Verification items for the finished model (mm, model axes). A direction names the side the tool comes from. Give positions to 0.01 mm unless a question says otherwise; leave off trailing zeros. Order: outer loops, then holes, each group sorted by start corner. A loop starts at its lowest first (then second) coordinate and runs counter-clockwise, first axis right, second up. Notation, with made-up numbers: (39, 80.5) -> (91, 80.5) arc R13 cw to (91, 98.5) -> close; hole circle Ø3 at (12, 55.5). An arc over 180 degrees is marked (long way). Return JSON: item names as keys, results as strings. Group by question number.
(1) Cross-section at A-A on y = -11.5. State how many separate pieces and enclosed holes the cut face has, then the cut area to 3 significant figures.
(2) Thickness scan on line 1 along Z through (x, y) = (-10, -8.25); line 2 along Y through (x, z) = (5.5, 5); line 3 along X through (y, z) = (-8.5, 3.5). Record the ranges inside material, lowest first.
(3) Cross-section at B-B on x = 9. Enter the section's corners in (y, z), then the cut area to 3 significant figures.
(4) Depth check by flat-ended pin: pin 1 Ø4 at (x, z) = (9.5, 0.5) entering from +Y; pin 2 Ø5 at (x, y) = (5, -5.5) entering from -Z; pin 3 Ø0.8 at (x, z) = (7.5, -0.5) entering from -Y; pin 4 Ø7 at (x, z) = (-8, -0.5) entering from -Y. Enter the tip coordinate at first touch or a pass-through.
(5) Cross-section at D-D on y = -6. Enter the section's corners in (x, z) (3 decimals), then the cut area to 3 significant figures.
(6) Cross-section at C-C on z = 0. Enter the section's corners in (x, y), then the cut area to 3 significant figures.
(7) Release check for a two-part mould opening along X. For faces 4 (the face through (4.5, -6.4, -1.7)), 5 (the face through (10, -7, -0.8)), 6 (the face through (12.2, -7, -2)) record: pulls with the +X half, pulls with the -X half, needs draft (parallel to the pull), parting line crosses it, or undercut.
(8) Tool access check on faces 1 (the face through (0, -3, 5)), 2 (the face through (-11, -7, 3.175)), 3 (the face through (8.342, -0.456, 0.355)). Record the directions out of +Z, -Z, +X, -X, +Y, -Y that give a thin tool (end or side, any length) a straight path to the whole face; none if there is none.
from build123d import *

# Parameters (mm, degrees)
SKETCH_2_R          = 0.75
EXTRUDE_1_DEPTH     = 1.5
CUT_EXTRUDE_1_DEPTH = 1.5
EXTRUDE_2_DEPTH     = 2.8
SKETCH_5_R          = 0.3
EXTRUDE_3_DEPTH     = 4.6


with BuildPart() as part:
    # 草图1 → 旋转1 (revolve)
    with BuildSketch(Plane.XY, mode=Mode.PRIVATE) as revolve_1_sk:
        Polygon((8.35, -5.5), (8.35, -6.4), (4.4, -6.4), (4.4, 0), (8.35, 0), (8.35, -0.9), (5, -0.9), (5, -5.5), align=None)
    revolve(revolve_1_sk.sketch.rotate(Axis((0, -3.284222298, 0), (0, 1, 0)), 90), axis=Axis((0, -3.284222298, 0), (0, 1, 0)))

    # 草图2 → 凸台-拉伸1 (add)
    with BuildSketch(Plane(origin=(0, 0, 0), x_dir=(1, 0, 0), z_dir=(0, 1, 0))):
        with Locations(Location((6, 0, 0), (0, 0, 270))):
            Circle(SKETCH_2_R)
    extrude(amount=EXTRUDE_1_DEPTH)

    # 草图3 → 切除-拉伸1 (cut)
    with BuildSketch(Plane(origin=(0, 0, 0), x_dir=(1, 0, 0), z_dir=(0, 1, 0))):
        with BuildLine():
            Line((-7.078375357, -0.851310072), (-10.983685898, -0.851310072))
            ThreePointArc((-10.983685898, -0.851310072), (-11.834995971, 0), (-10.983685898, 0.851310072))
            Line((-10.983685898, 0.851310072), (-7.078375357, 0.851310072))
            ThreePointArc((-7.078375357, 0.851310072), (-6.227065284, 0), (-7.078375357, -0.851310072))
        make_face()
    extrude(amount=-CUT_EXTRUDE_1_DEPTH, mode=Mode.SUBTRACT)

    # 草图4 → 凸台-拉伸2 (add)
    with BuildSketch(Plane(origin=(0, -5.5, 0), x_dir=(1, 0, 0), z_dir=(0, 1, 0))):
        with BuildLine():
            Line((-10.75, 4.8), (-6, 4.8))
            Line((-6, 4.8), (-6, -4.8))
            Line((-6, -4.8), (-10.75, -4.8))
            Line((-10.75, -4.8), (-10.75, -3.175))
            Line((-10.75, -3.175), (-12.2, -3.175))
            Line((-12.2, -3.175), (-12.2, -0.8))
            Line((-12.2, -0.8), (-7.078375357, -0.8))
            ThreePointArc((-7.078375357, -0.8), (-6.278375357, 0), (-7.078375357, 0.8))
            Line((-7.078375357, 0.8), (-12.2, 0.8))
            Line((-12.2, 0.8), (-12.2, 3.175))
            Line((-12.2, 3.175), (-10.75, 3.175))
            Line((-10.75, 3.175), (-10.75, 4.8))
        make_face()
        with BuildLine():
            Line((12.2, 3.175), (12.2, 0.8))
            Line((12.2, 0.8), (7.078375357, 0.8))
            ThreePointArc((7.078375357, 0.8), (6.278375357, 0), (7.078375357, -0.8))
            Line((7.078375357, -0.8), (12.2, -0.8))
            Line((12.2, -0.8), (12.2, -3.175))
            Line((12.2, -3.175), (10.75, -3.175))
            Line((10.75, -3.175), (10.75, -4.8))
            Line((10.75, -4.8), (6, -4.8))
            Line((6, -4.8), (6, 4.8))
            Line((6, 4.8), (10.75, 4.8))
            Line((10.75, 4.8), (10.75, 3.175))
            Line((10.75, 3.175), (12.2, 3.175))
        make_face()
    extrude(amount=-EXTRUDE_2_DEPTH)

    # 草图5 → 凸台-拉伸3 (add)
    with BuildSketch(Plane.XZ.offset(8.3)):
        with Locations(Location((-10.75, -1.75, 0), (0, 0, 90))):
            Circle(SKETCH_5_R)
        with Locations(Location((-7.25, -1.75, 0), (0, 0, 90))):
            Circle(SKETCH_5_R)
        with Locations(Location((-9, -3.5, 0), (0, 0, 90))):
            Circle(SKETCH_5_R)
        with Locations(Location((-9, 3.5, 0), (0, 0, 90))):
            Circle(SKETCH_5_R)
        with Locations(Location((-10.75, 1.75, 0), (0, 0, 90))):
            Circle(SKETCH_5_R)
        with Locations(Location((-7.25, 1.75, 0), (0, 0, 90))):
            Circle(SKETCH_5_R)
        with Locations(Location((7.25, 1.75, 0), (0, 0, 90))):
            Circle(SKETCH_5_R)
        with Locations(Location((10.75, 1.75, 0), (0, 0, 90))):
            Circle(SKETCH_5_R)
        with Locations(Location((10.75, -1.75, 0), (0, 0, 90))):
            Circle(SKETCH_5_R)
        with Locations(Location((7.25, -1.75, 0), (0, 0, 90))):
            Circle(SKETCH_5_R)
        with Locations(Location((9, -3.5, 0), (0, 0, 90))):
            Circle(SKETCH_5_R)
        with Locations(Location((9, 3.5, 0), (0, 0, 90))):
            Circle(SKETCH_5_R)
    extrude(amount=EXTRUDE_3_DEPTH)


solid = part.part
Verdict:
{
 "1": {"separate pieces": "12", "enclosed holes": "0", "area": "3.39 mm²"},
 "2": {"line 1": "-4.8 to -0.8, 0.8 to 4.8", "line 2": "-6.4 to -5.5, -0.9 to 0", "line 3": "-9.3 to -8.7, 8.7 to 9.3"},
 "3": {"outline": "(-12.9, -3.8) -> (-8.3, -3.8) -> (-8.3, -4.8) -> (-5.5, -4.8) -> (-5.5, -0.8) -> (-8.3, -0.8) -> (-8.3, -3.2) -> (-12.9, -3.2) -> close; (-12.9, 3.2) -> (-8.3, 3.2) -> (-8.3, 0.8) -> (-5.5, 0.8) -> (-5.5, 4.8) -> (-8.3, 4.8) -> (-8.3, 3.8) -> (-12.9, 3.8) -> close", "area": "27.9 mm²"},
 "4": {"pin 1": "y = 0", "pin 2": "z = -7.97", "pin 3": "y = -8.3", "pin 4": "y = -12.9"},
 "5": {"outline": "(-12.2, -3.175) -> (-10.75, -3.175) -> (-10.75, -4.8) -> (-6.832, -4.8) arc R8.35 ccw to (6.832, -4.8) -> (10.75, -4.8) -> (10.75, -3.175) -> (12.2, -3.175) -> (12.2, -0.8) -> (8.312, -0.8) arc R8.35 ccw to (8.312, 0.8) -> (12.2, 0.8) -> (12.2, 3.175) -> (10.75, 3.175) -> (10.75, 4.8) -> (6.832, 4.8) arc R8.35 ccw to (-6.832, 4.8) -> (-10.75, 4.8) -> (-10.75, 3.175) -> (-12.2, 3.175) -> (-12.2, 0.8) -> (-8.312, 0.8) arc R8.35 ccw to (-8.312, -0.8) -> (-12.2, -0.8) -> close; hole circle Ø8.8 at (0, 0)", "area": "220 mm²"},
 "6": {"outline": "(-8.35, -6.4) -> (-6.28, -6.4) -> (-6.28, -8.3) -> (-6, -8.3) -> (-6, -6.4) -> (-4.4, -6.4) -> (-4.4, 0) -> (-6.23, 0) -> (-6.23, -0.9) -> (-5, -0.9) -> (-5, -5.5) -> (-8.35, -5.5) -> close; (4.4, -6.4) -> (6, -6.4) -> (6, -8.3) -> (6.28, -8.3) -> (6.28, -6.4) -> (8.35, -6.4) -> (8.35, -5.5) -> (5, -5.5) -> (5, -0.9) -> (8.35, -0.9) -> (8.35, 0) -> (6.75, 0) -> (6.75, 1.5) -> (5.25, 1.5) -> (5.25, 0) -> (4.4, 0) -> close", "area": "21.1 mm²"},
 "7": {"face 4": "undercut", "face 5": "needs draft", "face 6": "pulls with the +X half"},
 "8": {"face 1": "none", "face 2": "+Z, -X, +Y, -Y", "face 3": "+Y"}
}
